from build123d import *


with BuildPart() as part:
    # Sketch1 → Revolve2 (revolve)
    with BuildSketch(Plane(origin=(0, 0, 0), x_dir=(0, 0, -1), z_dir=(1, 0, 0)), mode=Mode.PRIVATE) as revolve2_sk:
        Polygon((0, 0), (0, 3), (12, 3), (12, 4.25), (101, 4.25), (101, 3), (113, 3), (113, 0), align=None)
    revolve(revolve2_sk.sketch.rotate(Axis((0, 0, 0), (0, 0, -1)), 90), axis=Axis((0, 0, 0), (0, 0, -1)))


solid = part.part
Could you check a few things on this model? Use its own coordinates, in mm. A direction names the side the tool comes from. Give positions to 0.01 mm unless a question says otherwise; leave off trailing zeros. Write each loop counter-clockwise with the first axis right and the second up, starting at its lowest first coordinate (ties: lowest second). Pieces come first, ordered by that corner, then holes. Notation, with made-up numbers: (31, -36.75) - (54, -36.75) arc R27 ccw to (54, -2.75) - close; hole circle Ø5 at (45.5, 36.5). An arc over 180 degrees is marked (long way). Use CSV: the item, a comma, the result in double quotes. Start each with the question number.
Item 1: I want a section at A-A, the plane x = 0. Please give me the cut outline in (y, z).
Item 2: I want a section at C-C, the plane z = -26.5. Please give me the cut outline in (x, y), then the cut area to 3 significant figures.
Item 3: If I drill on line 1 along Y through (x, z) = (-3, -67); line 2 along Z through (x, y) = (-3, 2); line 3 along Y through (x, z) = (-1.25, -27), over which ranges is the centre line in solid material (lowest first)?
Item 4: I'm going to push flat-ended pins straight in: pin 1 (5 mm diameter, centred on y = 1, z = -42.5, fed in from -X); pin 2 (3 mm diameter, centred on y = 2.5, z = -27.5, fed in from +X); pin 3 (1.5 mm diameter, centred on y = -2.5, z = -15.5, fed in from +X). Where does each tip first touch, or does it pass through?
Item 5: For faces 1 (the face through (2.86, -0.9, -107.08)), 2 (the face through (0, 0, 0)), 3 (the face through (2.86, -0.9, -6.08)), which set-ups out of +Z, -Z, +X, -X, +Y, -Y let a thin tool reach every point of the face, with its end or its side?
Findings:
1,outline,"(-4.25, -101) - (-3, -101) - (-3, -113) - (3, -113) - (3, -101) - (4.25, -101) - (4.25, -12) - (3, -12) - (3, 0) - (-3, 0) - (-3, -12) - (-4.25, -12) - close"
2,outline,"circle Ø8.5 at (0, 0)"
2,area,"56.7 mm2"
3,line 1,"y = -3.01 to 3.01"
3,line 2,"z = -101 to -12"
3,line 3,"y = -4.06 to 4.06"
4,pin 1,"stops at x = -4.25"
4,pin 2,"stops at x = 4.13"
4,pin 3,"stops at x = 3.87"
5,face 1,"-Z"
5,face 2,"+Z, +X, -X, +Y, -Y"
5,face 3,"+Z"
